Work out the finished part from the listing and answer in its coordinate system (mm). A direction names the side the tool comes from. Coordinates: 2 decimals unless noted, no trailing zeros. Loops run counter-clockwise (first coordinate to the right, second up) from the corner with the lowest first, then second, coordinate; pieces in that order, holes last. Notation, with made-up numbers: (44.5, 8) -> (89.5, 8) arc R23 cw to (89.5, 37) -> close; hole circle Ø6 at (18.25, 12.5). An arc over 180 degrees is marked (long way). Answer as CSV lines item,"result".
Autodesk Inventor part; units mm, degrees
ref_plane "工作平面1" through (14, 0, 0) normal (1, 0, 0) x (0, 1, 0)
ref_plane "XZ Plane" through (0, 0, 0) normal (0, 1, 0) x (-1, 0, 0)
ref_plane "XY Plane" through (0, 0, 0) normal (0, 0, 1) x (1, 0, 0)
sketch "草图1" plane through (0, 0, 0) normal (0, 0, 1) x (1, 0, 0)
  line L0 (0, 0) -> (0, 4)
  line L1 (0, 4) -> (12, 4)
  line L2 (12, 4) -> (12, 3)
  line L3 (12, 3) -> (14, 3)
  line L4 (14, 3) -> (14, 5)
  line L5 (14, 5) -> (72.6225, 5)
  line L6 (72.6225, 5) -> (76, 10.85)
  line L7 (76, 10.85) -> (102, 8.25)
  line L8 (102, 8.25) -> (102, 0)
  line L9 (102, 0) -> (0, 0)
  dimension "d0" = 60
  dimension "d1" = 102
  dimension "d2" = 14
  dimension "d3" = 5
  dimension "d4" = 8.25
  dimension "d5" = 2
  dimension "d6" = 3
  dimension "d7" = 4
  dimension "d8" = 26
  dimension "d31" = 10.85
  dimension "d32" = 5.711
revolve "旋转1" add sketch "草图1" angle 360 about axis through (102, 0, 0) along (-1, 0, 0)
sketch "草图2" plane through (0, 0, 0) normal (0, 0, 1) x (1, 0, 0)
  line L0 (76, -10.85) -> (76, 10.85)
  line L1 (102, -8.25) -> (102, 8.25)
  line L2 (102, -8.25) -> (102, 8.25)
  line L3 (102, 0) -> (76, 0)
  line L4 (76, -10.85) -> (76, 10.85)
  circle A0 centre (86.5, 0) radius 5
  point P0 (0, 0)
  dimension "d10" = 10
  dimension "d11" = 15.5
extrude "拉伸1" cut sketch "草图2" against normal through all
sketch "草图3" plane through (0, 0, 0) normal (0, 0, 1) x (1, 0, 0)
  line L0 (76, -10.85) -> (76, 10.85)
  line L1 (102, -8.25) -> (102, 8.25)
  line L2 (102, -8.25) -> (102, 8.25)
  line L3 (102, -5) -> (80, -5)
  line L4 (80, -5) -> (76, 0)
  line L5 (76, 0) -> (102, 0)
  point P0 (0, 0)
  point P1 (86.7551, 4.9935)
  dimension "d14" = 5
  dimension "d15" = 22
revolve "旋转2" cut sketch "草图3" angle 360 about axis through (76, 0, 0) along (1, 0, 0)
thread "螺纹1"
ref_plane "工作平面1" through (14, 0, 0) normal (1, 0, 0) x (0, 1, 0)
sketch "草图4" plane through (14, 0, 0) normal (1, 0, 0) x (0, 1, 0)
  circle A0 centre (0, 0) radius 5
  line L0 (0, 5) -> (-5, 0)
  circle A1 centre (0, 0) radius 5
  line L1 (0, 5) -> (5, 0)
  point P0 (5, 0)
  dimension "d26" = 10
extrude "拉伸2" cut sketch "草图4" along normal blind 15 contours L1 A0 | L0 A0
chamfer "倒角3" distance 1.5 angle 45 2 edges at (0, -4, 0) (102, 5, 0)
properties part number "2-阀门" material "不锈钢"
(1) A cutting plane is placed at A-A, the plane x = 48. Write down the section's boundary in (y, z).
Computed values:
outline,"circle Ø10 at (0, 0)"
(2) A cutting plane is placed at C-C, the plane x = 86.5. Write down the section's boundary in (y, z).
Computed values:
outline,"(-5, -8.43) -> (-5, 0) arc R5 cw to (5, 0) -> (5, -8.43) arc R9.8 ccw (long way) to start"
(3) A cutting plane is placed at B-B, the plane x = 20. Write down the section's boundary in (y, z), and give its area (3 significant figures).
Computed values:
outline,"(-5, 0) arc R5 ccw to (5, 0) -> (0, 5) -> close"
area,"64.3 mm2"
(4) Which of the six approach directions +Z, -Z, +X, -X, +Y, -Y give full straight-line access (tool end or side, diameter ignored) to faces 1 (the face through (21, -2, 3)), 2 (the face through (82.815, 3.379, -6.223)), 3 (the face through (6.824, -0.867, -3.905)), 4 (the face through (12, 1, -3))?
Computed values:
face 1,"+Z, -Y"
face 2,"-Z"
face 3,"-X"
face 4,"none"
(5) Consider line 1 along Z through (x, y) = (94.5, 0); line 2 along X through (y, z) = (-4.25, -5.25); line 3 along Y through (x, z) = (93, 0). Determine where each line is inside the solid, lowest interval first.
Computed values:
line 1,"-9 to -5, 5 to 9"
line 2,"73.64 to 83.87, 89.13 to 102"
line 3,"-9.15 to -5, 5 to 9.15"
(6) Flat-ended cylindrical pins translate along their axes: pin 1 Ø12 at (x, z) = (29.5, 0) entering from -Y; pin 2 Ø3 at (x, z) = (77.5, 7.5) entering from -Y; pin 3 Ø9 at (x, y) = (86.5, 0) entering from -Z. Find the tip coordinate at first contact, or state that the pin passes through.
Computed values:
pin 1,"y = -5"
pin 2,"y = -8.88"
pin 3,"z = 2.18"
(7) For a pull along Z with two mould halves and no side action, classify faces 5 (the face through (72.834, 2.476, -4.761)), 6 (the face through (0, 0, 0)), 7 (the face through (90.106, 0.651, 4.957)) as pulls with the +Z half, pulls with the -Z half, needs draft (parallel to the pull), parting line crosses it, or undercut.
Computed values:
face 5,"parting line crosses it"
face 6,"needs draft"
face 7,"undercut"
